Autodesk Fusion 360 part; units mm, degrees
sketch "Base_Surface" plane through (0, 0, 0) normal (0, 0, 1) x (1, 0, 0)
  line L0 (-100, 0) -> (-100, 50)
  line L1 (-100, 50) -> (-2.5, 50)
  line L2 (-2.5, 50) -> (-2.5, 45)
  arc A0 (-2.5, 45) -> (2.5, 45) centre (0, 45) ccw
  line L3 (2.5, 45) -> (2.5, 50)
  line L4 (2.5, 50) -> (100, 50)
  line L5 (100, 50) -> (100, 0)
  line L6 (-100, 0) -> (100, 0) construction
  line L7 (-100, 42.5) -> (100, 42.5) construction
  line L8 (0, 0) -> (0, 45) construction
  line L9 (-100, 0) -> (-100, -50)
  line L10 (-100, -50) -> (-2.5, -50)
  line L11 (2.5, -50) -> (100, -50)
  line L12 (100, -50) -> (100, 0)
  line L13 (2.5, -45) -> (2.5, -50)
  arc A1 (2.5, -45) -> (-2.5, -45) centre (0, -45) ccw
  line L14 (-2.5, -50) -> (-2.5, -45)
  dimension "Total_Width" = 200
  dimension "Notch_Radius" = 2.5
  dimension "Notch_Height" = 7.5
  dimension "Total_Height" = 100
extrude "Extrude1" add sketch "Base_Surface" along normal mid plane 10
Check sheet for the modelled part. Datum: model origin and axes. Units: mm. A direction names the side the tool comes from. Round coordinates to 2 decimals unless told otherwise and drop trailing zeros. Write each loop counter-clockwise with the first axis right and the second up, starting at its lowest first coordinate (ties: lowest second). Pieces come first, ordered by that corner, then holes. Notation, with made-up numbers: (24.5, 65.25) -> (51.5, 65.25) arc R17 cw to (51.5, 70.25) -> close; hole circle Ø10 at (28, -3). An arc over 180 degrees is marked (long way). Put each result on its own line as item: value.
(1) Mould release check, pull along X, two halves, no side actions. Record for faces 4 (the face through (0.1, 42.5, -0.1)), 5 (the face through (51, 50, 0)), 6 (the face through (100, 1, 0)): released by +X, released by -X, zero draft, split by the parting line, or undercut.
Values found:
face 4: undercut
face 5: zero draft
face 6: released by +X
(2) Material ranges on line 1 (X direction, y = 43, z = -4); line 2 (Y direction, x = 1, z = 0.5), recorded low to high.
Values found:
line 1: x = -100 to -1.5, 1.5 to 100
line 2: y = -42.71 to 42.71
(3) Tool access check on faces 1 (the face through (51, -50, 0)), 2 (the face through (2.5, 47, 0)), 3 (the face through (-2.5, -48, 0)). Record the directions out of +Z, -Z, +X, -X, +Y, -Y that give a thin tool (end or side, any length) a straight path to the whole face; none if there is none.
Values found:
face 1: +Z, -Z, +X, -X, -Y
face 2: +Z, -Z, +Y
face 3: +Z, -Z, -Y
(4) Sectioned sample at A-A (x = 0). Enter the section's corners in (y, z), plus the area to 3 significant figures.
Values found:
outline: (-42.5, -5) -> (42.5, -5) -> (42.5, 5) -> (-42.5, 5) -> close
area: 850 mm^2
